For this review, take the finished solid that the model builds, in its own axes (mm). Round coordinates to 2 decimals unless told otherwise and drop trailing zeros. Loops run counter-clockwise (first coordinate to the right, second up) from the corner with the lowest first, then second, coordinate; pieces in that order, holes last.
```python
from build123d import *

# Parameters (mm, degrees)
SKETCH_1_W          = 10
SKETCH_1_H          = 10
SKETCH_1_W_2        = 7
SKETCH_1_H_2        = 7
EXTRUDE_1_DEPTH     = 750
SKETCH_2_R          = 2.15
CUT_EXTRUDE_1_DEPTH = 751.083328704


with BuildPart() as part:
    # ｽｹｯﾁ1 → 押し出し-薄板1 (new body)
    with BuildSketch(Plane(origin=(0, 0, 0), x_dir=(0, 0, -1), z_dir=(1, 0, 0))):
        Rectangle(SKETCH_1_W, SKETCH_1_H)
        Rectangle(SKETCH_1_W_2, SKETCH_1_H_2, mode=Mode.SUBTRACT)
    extrude(amount=EXTRUDE_1_DEPTH)

    # ｽｹｯﾁ2 → ｶｯﾄ - 押し出し1 (cut, through all)
    with BuildSketch(Plane(origin=(0, 5, 0), x_dir=(1, 0, 0), z_dir=(0, 1, 0))):
        with Locations(Location((745, 0, 0), (0, 0, 270))):
            Circle(SKETCH_2_R)
        with Locations(Location((5, 0, 0), (0, 0, 270))):
            Circle(SKETCH_2_R)
        with Locations(Location((505.5, 0, 0), (0, 0, 270))):
            Circle(SKETCH_2_R)
        with Locations(Location((244.5, 0, 0), (0, 0, 270))):
            Circle(SKETCH_2_R)
        with Locations(Location((637.5, 0, 0), (0, 0, 270))):
            Circle(SKETCH_2_R)
        with Locations(Location((112.5, 0, 0), (0, 0, 270))):
            Circle(SKETCH_2_R)
        with Locations(Location((375, 0, 0), (0, 0, 270))):
            Circle(SKETCH_2_R)
    extrude(amount=-CUT_EXTRUDE_1_DEPTH, mode=Mode.SUBTRACT)


solid = part.part
```
(1) Add section A-A (y = 2). Give the boundary of the cut face in (x, z), plus the area to 3 significant figures.
(2) Add section C-C (z = 0). Give the number of separate pieces and of enclosed holes in the cut face, plus the area to 3 significant figures.
(3) For L1, parallel to Z at x = 252.5, y = -3; L2, parallel to Z at x = 637.5, y = 4.2, list the stretches that pass through material, from the lowest coordinate up.
(4) Add section B-B (x = 396). Give the boundary of the cut face in (y, z), plus the area to 3 significant figures.
Outcome:
1. outline: (0, -5) - (750, -5) - (750, -3.5) - (0, -3.5) - close; (0, 3.5) - (750, 3.5) - (750, 5) - (0, 5) - close
1. area: 2,250 mm2
2. separate pieces: 16
2. enclosed holes: 0
2. area: 2,160 mm2
3. L1: z = -5 to -3.5, 3.5 to 5
3. L2: z = -5 to -2.15, 2.15 to 5
4. outline: (-5, -5) - (5, -5) - (5, 5) - (-5, 5) - close; hole (-3.5, -3.5) - (3.5, -3.5) - (3.5, 3.5) - (-3.5, 3.5) - close
4. area: 51.0 mm2
